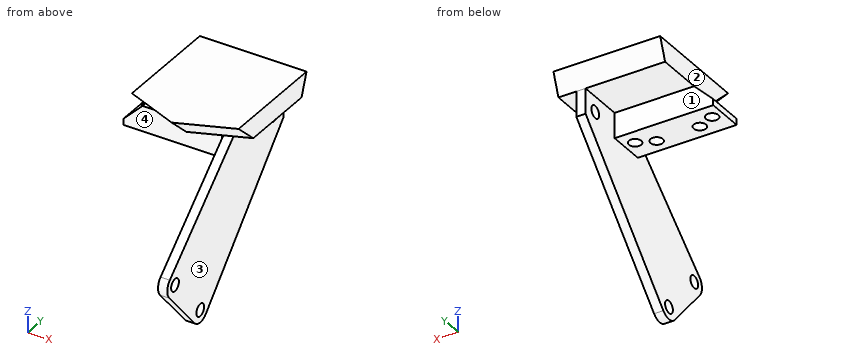
from build123d import *

# Parameters (mm, degrees)
RESSALTO_EXTRUS_O4_DEPTH = 7
CHANFRO1_SIZE            = 7
CHANFRO2_SIZE2           = 7
CHANFRO2_SIZE            = 2.54779164
RESSALTO_EXTRUS_O5_DEPTH = 12
ESBO_O13_R               = 2
CORTE_EXTRUS_O1_DEPTH    = 5
ESBO_O14_R               = 2
RESSALTO_EXTRUS_O6_DEPTH = 3


with BuildPart() as part:
    # Esboço10 → Ressalto-extrusão4 (new body)
    with BuildSketch(Plane.XY):
        Polygon((-17.3, -17.5), (0, -24.5), (17.3, -17.5), (17.3, 17.5), (-17.3, 17.5), align=None)
    extrude(amount=-RESSALTO_EXTRUS_O4_DEPTH)

    # Chanfro1
    chanfro1_edges = [part.edges().sort_by_distance(p)[0] for p in [
        (-8.65, -21, -7),
        (8.65, -21, -7),
    ]]
    chamfer(chanfro1_edges, length=CHANFRO1_SIZE - 0.0001)  # a hair under: the kernel refuses the full size

    # Chanfro2
    chanfro2_edges = [part.edges().sort_by_distance(p)[0] for p in [
        (0, 17.5, -7),
    ]]
    chanfro2_side = [part.faces().sort_by_distance(p)[0] for p in [
        (0, 17.449044167, -7),
    ]]
    chamfer(chanfro2_edges, length=CHANFRO2_SIZE - 0.0001, length2=CHANFRO2_SIZE2 - 0.0001, reference=chanfro2_side[0])  # a hair under: the kernel refuses the full size

    # Esboço12 → Ressalto-extrusão5 (add)
    with BuildSketch(Plane(origin=(0, 0, 0), x_dir=(1, 0, 0), z_dir=(0, 1, 0))):
        Polygon((-17.3, 7), (-23.5, 13.2), (-23.5, 15.2), (8.5, 15.2), (8.5, 7), align=None)
    extrude(amount=-RESSALTO_EXTRUS_O5_DEPTH)

    # Esboço13 → Corte-extrusão1 (cut)
    with BuildSketch(Plane(origin=(0, 0, -15.2), x_dir=(-1, 0, 0), z_dir=(0, 0, -1))):
        with Locations((0.5, -7.397915762)):
            Circle(ESBO_O13_R)
        with Locations((-5, -5)):
            Circle(ESBO_O13_R)
        with Locations(Location((20, -5, 0), (0, 0, 284.477512186))):
            Circle(ESBO_O13_R)
        with Locations(Location((14.5, -7.397915762, 0), (0, 0, 180))):
            Circle(ESBO_O13_R)
    extrude(amount=-CORTE_EXTRUS_O1_DEPTH, mode=Mode.SUBTRACT)

    # Esboço14 → Ressalto-extrusão6 (add)
    with BuildSketch(Plane(origin=(8.5, 0, 0), x_dir=(0, 0, -1), z_dir=(1, 0, 0))):
        with BuildLine():
            Line((57.743206586, -25.136637637), (15.2, 14.95220836))
            Line((15.2, 14.95220836), (7, 14.95220836))
            Line((7, 14.95220836), (7, -9.948687565))
            Line((7, -9.948687565), (37.010562028, -43.705471194))
            ThreePointArc((37.010562028, -43.705471194), (39.740206409, -45.039346135), (42.619722154, -44.070547971))
            Line((42.619722154, -44.070547971), (57.619722154, -31.070547971))
            ThreePointArc((57.619722154, -31.070547971), (58.999134172, -28.131013459), (57.743206586, -25.136637637))
        make_face()
        with Locations((12, 9.95220836)):
            Circle(ESBO_O14_R, mode=Mode.SUBTRACT)
        with Locations((55, -28.04779164)):
            Circle(ESBO_O14_R, mode=Mode.SUBTRACT)
        with Locations((40, -41.04779164)):
            Circle(ESBO_O14_R, mode=Mode.SUBTRACT)
    extrude(amount=RESSALTO_EXTRUS_O6_DEPTH)


solid = part.part
Verification items for the finished model (mm, model axes). Face numbers are marked on the shaded views. A direction names the side the tool comes from. Give positions to 0.01 mm unless a question says otherwise; leave off trailing zeros. Write each loop counter-clockwise with the first axis right and the second up, starting at its lowest first coordinate (ties: lowest second). Pieces come first, ordered by that corner, then holes.
(1) Material ranges on line 1 (Y direction, x = 5, z = -13.65); line 2 (Y direction, x = -10, z = -13); line 3 (X direction, y = -21.5, z = -34), recorded low to high.
(2) Access from +Z, -Z, +X, -X, +Y, -Y to the whole of each face (thin tool, end or side, straight path). Record for the marked faces 1, 2, 3 and 4.
(3) Gauge pin test, flat ends, axial feed: pin 1 (1 mm diameter, centred on y = -38, z = -42, fed in from +X); pin 2 (9 mm diameter, centred on x = -2.5, z = -12, fed in from -Y); pin 3 (4.5 mm diameter, centred on x = -15, y = -7, fed in from -Z). Record the tip position at first contact, or that the pin passes through.
(4) Cross-section at A-A (z = -40.5). Enter the section's corners in (x, y), plus the area to 3 significant figures.
(5) Cross-section at D-D (z = -4). Enter the section's corners in (x, y), plus the area to 3 significant figures.
Worked out:
1. line 1: y = -12 to -7, -3 to 0
1. line 2: y = -12 to 0
1. line 3: x = 8.5 to 11.5
2. face 1: -Z, -X, +Y
2. face 2: +Z, -X, +Y, -Y
2. face 3: -Z, +X, +Y, -Y
2. face 4: -Z, -X, -Y
3. pin 1: stops at x = 11.5
3. pin 2: stops at y = -12
3. pin 3: stops at z = -15.2
4. outline: (8.5, -45.02) - (11.5, -45.02) - (11.5, -42.98) - (8.5, -42.98) - close; (8.5, -39.11) - (11.5, -39.11) - (11.5, -8.89) - (8.5, -8.89) - close
4. area: 96.8 mm2
5. outline: (-17.3, -13.19) - (0, -20.19) - (17.3, -13.19) - (17.3, 16.04) - (-17.3, 16.04) - close
5. area: 1,130 mm2
